Work out the finished part from the listing and answer in its coordinate system (mm). A direction names the side the tool comes from. Coordinates: 2 decimals unless noted, no trailing zeros. Write each loop counter-clockwise with the first axis right and the second up, starting at its lowest first coordinate (ties: lowest second). Pieces come first, ordered by that corner, then holes. Notation, with made-up numbers: (-21.5, 66) - (37.5, 66) arc R22 cw to (37.5, 86) - close; hole circle Ø2 at (-34.5, 19). An arc over 180 degrees is marked (long way). Use one line per item in the form item = value. Start each with the question number.
Item 1: Consider probe 1 along Z at (x, y) = (-2, 4.6); probe 2 along Z at (x, y) = (2.5, 3.3); probe 3 along Z at (x, y) = (-10.5, 1.1). Determine where each line is inside the solid, lowest interval first.
Item 2: For faces 1 (the flat face through (-13, 2, -25)), 2 (the flat face through (-72, 3, -110)), 3 (the flat face through (-70, 2, -5)), determine the directions among +Z, -Z, +X, -X, +Y, -Y from which every point of the face is accessible in a straight line to the end or side of a thin tool.
Item 3: A cutting plane is placed at A-A (z = -75.5). Write down the section's boundary in (x, y), then the cut area to 3 significant figures.
Item 4: Given pin 1 (1.5 mm diameter, centred on x = -71.5, y = 3, fed in from +Z); pin 2 (1.6 mm diameter, centred on y = 2.5, z = -27, fed in from +X); pin 3 (2 mm diameter, centred on y = 3, z = -97.5, fed in from -X); pin 4 (12 mm diameter, centred on x = -30, z = -96.5, fed in from -Y), each flat-ended and moving along its own axis, determine where each tip first touches the part or whether it passes through.
Item 5: Determine the mould class of faces 4 (the flat face through (-60, 2, -21.5)), 5 (the flat face through (0, 2, -22)), 6 (the flat face through (-66, 2, -26.5)) for opening direction X: released by +X, released by -X, zero draft, split by the parting line, or undercut.
Autodesk Inventor part; units mm, degrees
ref_plane "Work Plane2" through (0, 0, 0) normal (0, -1, 0) x (1, 0, 0)
ref_plane "Work Plane3" through (0, 0, 0) normal (1, 0, 0) x (0, 0, -1)
ref_plane "Work Plane1" through (-70, 0, 0) normal (-1, 0, 0) x (0, 0, 1)
sketch "Sketch1" plane through (0, 0, 0) normal (0, 1, 0) x (-1, 0, 0)
  line L0 (0, -120) -> (70, -120)
  line L1 (70, 0) -> (0, 0)
  line L2 (0, 0) -> (0, -5)
  line L3 (0, -120) -> (0, -115)
  line L4 (0, -5) -> (0, -3.5)
  line L5 (0, -120) -> (0, -115)
  line L6 (70, 45) -> (70, 46.5)
  line L7 (70, -73.5) -> (70, -26.5)
  line L8 (70, -60) -> (70, -58.5)
  line L9 (70, -73.5) -> (70, -88.5)
  line L10 (0, -115) -> (0, -120)
  line L11 (70, -73.5) -> (70, -76.5)
  line L12 (0, -33.5) -> (0, -36.5)
  line L13 (0, -80) -> (0, -36.5)
  line L14 (0, -55) -> (0, -26.5)
  line L15 (0, -26.5) -> (8, -26.5)
  line L16 (8, -26.5) -> (8, -28.5)
  line L17 (8, -28.5) -> (13, -28.5)
  line L18 (13, -28.5) -> (13, -21.5)
  line L19 (13, -21.5) -> (8, -21.5)
  line L20 (8, -21.5) -> (8, -23.5)
  line L21 (8, -23.5) -> (0, -23.5)
  line L22 (13, -25) -> (57, -25)
  line L23 (70, -25) -> (70, -23.5)
  line L24 (70, -23.5) -> (62, -23.5)
  line L25 (62, -23.5) -> (62, -21.5)
  line L26 (62, -21.5) -> (57, -21.5)
  line L27 (57, -21.5) -> (57, -28.5)
  line L28 (57, -28.5) -> (62, -28.5)
  line L29 (62, -28.5) -> (62, -26.5)
  line L30 (62, -26.5) -> (70, -26.5)
  line L31 (0, 0) -> (0, -23.5)
  line L32 (0, -26.5) -> (0, -55)
  line L33 (0, -5) -> (0, -23.5)
  line L34 (0, -26.5) -> (0, -33.5)
  line L35 (0, -5) -> (0, -23.5)
  line L36 (0, -26.5) -> (0, -33.5)
  line L37 (0, 0) -> (0, -23.5)
  line L38 (0, -26.5) -> (0, -33.5)
  line L39 (70, 0) -> (70, -23.5)
  line L40 (70, -26.5) -> (70, -88.5)
  line L41 (0, -83.5) -> (0, -80)
  line L42 (0, -80) -> (0, -83.5)
  line L43 (70, -88.5) -> (70, -76.5)
  line L44 (13, -25) -> (0, -25)
  line L45 (0, -83.5) -> (0, -88.5)
  line L46 (0, -91.5) -> (0, -88.5)
  line L47 (70, -91.5) -> (70, -88.5)
  line L48 (0, -26.5) -> (0, -60)
  line L49 (0, -60) -> (70, -60)
  line L50 (0, -93.5) -> (8, -93.5)
  line L51 (8, -93.5) -> (8, -91.5)
  line L52 (8, -91.5) -> (13, -91.5)
  line L53 (13, -91.5) -> (13, -98.5)
  line L54 (13, -98.5) -> (8, -98.5)
  line L55 (8, -98.5) -> (8, -96.5)
  line L56 (8, -96.5) -> (0, -96.5)
  line L57 (13, -95) -> (57, -95)
  line L58 (70, -96.5) -> (62, -96.5)
  line L59 (62, -96.5) -> (62, -98.5)
  line L60 (62, -98.5) -> (57, -98.5)
  line L61 (57, -98.5) -> (57, -91.5)
  line L62 (57, -91.5) -> (62, -91.5)
  line L63 (62, -91.5) -> (62, -93.5)
  line L64 (62, -93.5) -> (70, -93.5)
  line L65 (0, -93.5) -> (0, -86.5)
  line L66 (0, -93.5) -> (0, -86.5)
  line L67 (0, -93.5) -> (0, -86.5)
  line L68 (0, -91.5) -> (0, -93.5)
  line L69 (0, -96.5) -> (0, -110)
  line L70 (0, -120) -> (0, -96.5)
  line L71 (0, -93.5) -> (0, -91.5)
  line L72 (70, -120) -> (70, -96.5)
  line L73 (70, -93.5) -> (70, -91.5)
  dimension "d70" = 120
  dimension "d115" = 5
  dimension "d116" = 7
  dimension "d117" = 5
  dimension "d119" = 8
  dimension "d120" = 2
  dimension "d121" = 5
  dimension "d123" = 25
  dimension "d124" = 1.5
  dimension "d125" = 1.5
  dimension "d126" = 1.5
  dimension "d127" = 1.5
  dimension "d128" = 35
  dimension "d130" = 70
  dimension "d131" = 8
  dimension "d132" = 2
ref_plane "Work Plane2" through (0, 0, 0) normal (0, -1, 0) x (1, 0, 0)
sketch "Sketch2" plane through (0, 0, 0) normal (0, -1, 0) x (1, 0, 0)
  point P0 (0, 0)
ref_plane "Work Plane3" through (0, 0, 0) normal (1, 0, 0) x (0, 0, -1)
sketch "Sketch3" plane through (0, 0, 0) normal (1, 0, 0) x (0, 0, -1)
  line L0 (0, 0) -> (10, 0)
  line L1 (10, 0) -> (10, 5)
  line L2 (10, 5) -> (20, 5)
  line L3 (20, 5) -> (20, 0)
  line L4 (20, 0) -> (10, 0)
  line L5 (20, 0) -> (30, 0)
  line L6 (30, 0) -> (30, 5)
  line L7 (30, 5) -> (40, 5)
  line L8 (40, 5) -> (40, 0)
  line L9 (40, 0) -> (30, 0)
  line L10 (40, 0) -> (80, 0)
  line L11 (80, 0) -> (80, 5)
  line L12 (80, 5) -> (90, 5)
  line L13 (90, 5) -> (90, 0)
  line L14 (90, 0) -> (100, 0)
  line L15 (100, 0) -> (100, 5)
  line L16 (100, 5) -> (110, 5)
  line L17 (110, 5) -> (110, 0)
  line L18 (110, 0) -> (100, 0)
  line L19 (90, 0) -> (80, 0)
  dimension "d46" = 10
  dimension "d47" = 5
  dimension "d48" = 10
  dimension "d49" = 10
  dimension "d50" = 10
  dimension "d75" = 5
  dimension "d76" = 10
  dimension "d77" = 10
  dimension "d78" = 5
  dimension "d79" = 10
  dimension "d129" = 40
ref_plane "Work Plane1" through (-70, 0, 0) normal (-1, 0, 0) x (0, 0, 1)
sketch "Sketch4" plane through (-70, 0, 0) normal (-1, 0, 0) x (0, 0, 1)
  line L0 (0, 0) -> (-10, 0)
  line L1 (-10, 0) -> (-10, 5)
  line L2 (-10, 5) -> (-20, 5)
  line L3 (-20, 5) -> (-20, 0)
  line L4 (-10, 0) -> (-20, 0)
  line L5 (-20, 0) -> (-30, 0)
  line L6 (-30, 0) -> (-30, 5)
  line L7 (-30, 5) -> (-40, 5)
  line L8 (-40, 5) -> (-40, 0)
  line L9 (-40, 0) -> (-30, 0)
  line L10 (-40, 5) -> (-40, 0)
  line L11 (-40, 0) -> (-80, 0)
  line L12 (-80, 0) -> (-80, 5)
  line L13 (-80, 5) -> (-90, 5)
  line L14 (-90, 5) -> (-90, 0)
  line L15 (-90, 0) -> (-80, 0)
  line L16 (-90, 0) -> (-100, 0)
  line L17 (-100, 0) -> (-100, 5)
  line L18 (-100, 5) -> (-110, 5)
  line L19 (-110, 5) -> (-110, 0)
  line L20 (-100, 0) -> (-110, 0)
  dimension "d58" = 10
  dimension "d59" = 5
  dimension "d60" = 10
  dimension "d61" = 10
  dimension "d62" = 10
  dimension "d80" = 40
  dimension "d81" = 10
  dimension "d82" = 10
  dimension "d83" = 10
extrude "Extrusion12" add sketch "Sketch1" along normal blind 5
extrude "Extrusion13" add sketch "Sketch3" along normal blind 5
extrude "Extrusion14" add sketch "Sketch4" along normal blind 5
properties part number "frontal"
Answer:
q1.probe_1 = -120 to -96.5, -93.5 to -26.5, -23.5 to 0
q1.probe_2 = -110 to -100, -90 to -80, -40 to -30, -20 to -10
q1.probe_3 = -120 to -98.5, -91.5 to -28.5, -21.5 to 0
q2.face_1 = +Y, -Y
q2.face_2 = -Z, -X, +Y, -Y
q2.face_3 = +Z, -X, +Y, -Y
q3.outline = (-70, 0) - (0, 0) - (0, 5) - (-70, 5) - close
q3.area = 350 mm²
q4.pin_1 = -10
q4.pin_2 = 0
q4.pin_3 = -70
q4.pin_4 = 0
q5.face_4 = undercut
q5.face_5 = released by +X
q5.face_6 = zero draft
